Could you check a few things on this model? Use its own coordinates, in mm. A direction names the side the tool comes from. Coordinates: 2 decimals unless noted, no trailing zeros. Loops run counter-clockwise (first coordinate to the right, second up) from the corner with the lowest first, then second, coordinate; pieces in that order, holes last. Notation, with made-up numbers: (16, -21.5) -> (58, -21.5) arc R15 cw to (58, -1.5) -> close; hole circle Ø2 at (-1, 16). An arc over 180 degrees is marked (long way). One line per question, with ' | ' between items.
from build123d import *

# Parameters (mm, degrees)
SKETCH1_W           = 500
SKETCH1_H           = 500
BOSS_EXTRUDE1_DEPTH = 3
CUT_EXTRUDE1_REACH  = 355.566
SKETCH3_R           = 4
SKETCH4_W           = 500
SKETCH4_H           = 500
SKETCH4_W_2         = 494
SKETCH4_H_2         = 494
BOSS_EXTRUDE2_DEPTH = 30
SKETCH5_W           = 494
SKETCH5_H           = 494
SKETCH5_W_2         = 394
SKETCH5_H_2         = 394
BOSS_EXTRUDE3_DEPTH = 3
CUT_EXTRUDE2_REACH  = 357.09
SKETCH6_R           = 6


with BuildPart() as part:
    # Sketch1 → Boss-Extrude1 (new body)
    with BuildSketch(Plane.XY):
        Rectangle(SKETCH1_W, SKETCH1_H)
    extrude(amount=BOSS_EXTRUDE1_DEPTH)

    # Sketch3 → Cut-Extrude1 (cut, up to next)
    with BuildSketch(Plane(origin=(0, 0, 0), x_dir=(-1, 0, 0), z_dir=(0, 0, -1)), mode=Mode.PRIVATE) as cut_extrude1_sk1:
        with Locations((50, 50)):
            Circle(SKETCH3_R)
    cut_extrude1_tool1 = extrude(cut_extrude1_sk1.sketch, amount=-CUT_EXTRUDE1_REACH, mode=Mode.PRIVATE) & part.part
    # Sketch3 → Cut-Extrude1 (cut, up to next)
    with BuildSketch(Plane(origin=(0, 0, 0), x_dir=(-1, 0, 0), z_dir=(0, 0, -1)), mode=Mode.PRIVATE) as cut_extrude1_sk2:
        with Locations((-50, 50)):
            Circle(SKETCH3_R)
    cut_extrude1_tool2 = extrude(cut_extrude1_sk2.sketch, amount=-CUT_EXTRUDE1_REACH, mode=Mode.PRIVATE) & part.part
    # Sketch3 → Cut-Extrude1 (cut, up to next)
    with BuildSketch(Plane(origin=(0, 0, 0), x_dir=(-1, 0, 0), z_dir=(0, 0, -1)), mode=Mode.PRIVATE) as cut_extrude1_sk3:
        with Locations((50, -50)):
            Circle(SKETCH3_R)
    cut_extrude1_tool3 = extrude(cut_extrude1_sk3.sketch, amount=-CUT_EXTRUDE1_REACH, mode=Mode.PRIVATE) & part.part
    # Sketch3 → Cut-Extrude1 (cut, up to next)
    with BuildSketch(Plane(origin=(0, 0, 0), x_dir=(-1, 0, 0), z_dir=(0, 0, -1)), mode=Mode.PRIVATE) as cut_extrude1_sk4:
        with Locations((-50, -50)):
            Circle(SKETCH3_R)
    cut_extrude1_tool4 = extrude(cut_extrude1_sk4.sketch, amount=-CUT_EXTRUDE1_REACH, mode=Mode.PRIVATE) & part.part
    add(cut_extrude1_tool1.solids().sort_by_distance((-50, 50, 0))[0], mode=Mode.SUBTRACT)
    add(cut_extrude1_tool2.solids().sort_by_distance((50, 50, 0))[0], mode=Mode.SUBTRACT)
    add(cut_extrude1_tool3.solids().sort_by_distance((-50, -50, 0))[0], mode=Mode.SUBTRACT)
    add(cut_extrude1_tool4.solids().sort_by_distance((50, -50, 0))[0], mode=Mode.SUBTRACT)

    # Sketch4 → Boss-Extrude2 (add)
    with BuildSketch(Plane.XY.offset(3)):
        Rectangle(SKETCH4_W, SKETCH4_H)
        Rectangle(SKETCH4_W_2, SKETCH4_H_2, mode=Mode.SUBTRACT)
    extrude(amount=BOSS_EXTRUDE2_DEPTH)

    # Sketch5 → Boss-Extrude3 (add)
    with BuildSketch(Plane.XY.offset(33)):
        Rectangle(SKETCH5_W, SKETCH5_H)
        Rectangle(SKETCH5_W_2, SKETCH5_H_2, mode=Mode.SUBTRACT)
    extrude(amount=-BOSS_EXTRUDE3_DEPTH)

    # Sketch6 → Cut-Extrude2 (cut, up to next)
    with BuildSketch(Plane.XY.offset(33), mode=Mode.PRIVATE) as cut_extrude2_sk1:
        with Locations((-223.5, 223.5)):
            Circle(SKETCH6_R)
    cut_extrude2_tool1 = extrude(cut_extrude2_sk1.sketch, amount=-CUT_EXTRUDE2_REACH, mode=Mode.PRIVATE) & part.part
    # Sketch6 → Cut-Extrude2 (cut, up to next)
    with BuildSketch(Plane.XY.offset(33), mode=Mode.PRIVATE) as cut_extrude2_sk2:
        with Locations((223.5, 223.5)):
            Circle(SKETCH6_R)
    cut_extrude2_tool2 = extrude(cut_extrude2_sk2.sketch, amount=-CUT_EXTRUDE2_REACH, mode=Mode.PRIVATE) & part.part
    # Sketch6 → Cut-Extrude2 (cut, up to next)
    with BuildSketch(Plane.XY.offset(33), mode=Mode.PRIVATE) as cut_extrude2_sk3:
        with Locations((223.5, -223.5)):
            Circle(SKETCH6_R)
    cut_extrude2_tool3 = extrude(cut_extrude2_sk3.sketch, amount=-CUT_EXTRUDE2_REACH, mode=Mode.PRIVATE) & part.part
    # Sketch6 → Cut-Extrude2 (cut, up to next)
    with BuildSketch(Plane.XY.offset(33), mode=Mode.PRIVATE) as cut_extrude2_sk4:
        with Locations((-223.5, -223.5)):
            Circle(SKETCH6_R)
    cut_extrude2_tool4 = extrude(cut_extrude2_sk4.sketch, amount=-CUT_EXTRUDE2_REACH, mode=Mode.PRIVATE) & part.part
    add(cut_extrude2_tool1.solids().sort_by_distance((-223.5, 223.5, 33))[0], mode=Mode.SUBTRACT)
    add(cut_extrude2_tool2.solids().sort_by_distance((223.5, 223.5, 33))[0], mode=Mode.SUBTRACT)
    add(cut_extrude2_tool3.solids().sort_by_distance((223.5, -223.5, 33))[0], mode=Mode.SUBTRACT)
    add(cut_extrude2_tool4.solids().sort_by_distance((-223.5, -223.5, 33))[0], mode=Mode.SUBTRACT)


solid = part.part
1) I need wall thicknesses on line 1 along Y through (x, z) = (50, 2); line 2 along Z through (x, y) = (203, -32.5); line 3 along X through (y, z) = (195.5, 10.5). Which ranges of each line are inside material? Lowest first, please. Write a range as from..to.
Data:
line 1: -250..-54, -46..46, 54..250 | line 2: 0..3, 30..33 | line 3: -250..-247, 247..250
2) I'm going to push flat-ended pins straight in: pin 1 Ø11 at (x, y) = (223.5, 223.5) entering from +Z; pin 2 Ø6.5 at (x, y) = (-50, 50) entering from -Z. Where does each tip first touch, or does it pass through?
Data:
pin 1: z = 3 | pin 2: through
3) If we section it at C-C on x = -97: Please give me the cut outline in (y, z), and give its area (3 significant figures).
Data:
outline: (-250, 0) -> (250, 0) -> (250, 33) -> (197, 33) -> (197, 30) -> (247, 30) -> (247, 3) -> (-247, 3) -> (-247, 30) -> (-197, 30) -> (-197, 33) -> (-250, 33) -> close | area: 1,980 mm²
4) On a 3-axis mill with a long thin cutter (end or side, diameter ignored), from which of +Z, -Z, +X, -X, +Y, -Y can I reach the whole of each face in a straight line? I mean faces 4 (the face through (-3, 250, 16)), 5 (the face through (-217.777, 225.302, 31.521)), 6 (the face through (-3, 3, 3)). Say none if no direction works.
Data:
face 4: +Z, -Z, +X, -X, +Y | face 5: +Z | face 6: none
5) We'd pull the mould along Z, two halves only. Please class faces 1 (the face through (-217.777, -221.698, 31.521)), 2 (the face through (-247, -3, 16)), 3 (the face through (-3, 4, 0)): pulls with the +Z half, pulls with the -Z half, needs draft (parallel to the pull), parting line crosses it, or undercut.
Data:
face 1: needs draft | face 2: undercut | face 3: pulls with the -Z half
6) If we section it at B-B on z = 14: Please give me the cut outline in (x, y).
Data:
outline: (-250, -250) -> (250, -250) -> (250, 250) -> (-250, 250) -> close; hole (-247, -247) -> (247, -247) -> (247, 247) -> (-247, 247) -> close
7) If we section it at A-A on x = 211: Please give me the cut outline in (y, z).
Data:
outline: (-250, 0) -> (250, 0) -> (250, 33) -> (-250, 33) -> close; hole (-247, 3) -> (247, 3) -> (247, 30) -> (-247, 30) -> close
